For this review, take the finished solid that the model builds, in its own axes (mm). Round coordinates to 2 decimals unless told otherwise and drop trailing zeros. Loops run counter-clockwise (first coordinate to the right, second up) from the corner with the lowest first, then second, coordinate; pieces in that order, holes last. Notation, with made-up numbers: (-20.75, 28) -> (19.25, 28) arc R26 cw to (19.25, 46) -> close; hole circle Ø1 at (-9, -23.75). An arc over 180 degrees is marked (long way). One line per question, with ' | ' between items. Start each with the question number.
1. Consider section B-B (z = -61). Write out the cut boundary in (x, y).
2. Consider section A-A (z = -15). Write out the cut boundary in (x, y), and give its area (4 significant figures).
3. For pin 1 Ø4 at (x, z) = (0, -15) entering from +Y, flat-tipped, find the tip position at first contact; note if it passes through.
4. Consider section C-C (y = 3.25). Count the separate pieces of the cut face and the enclosed holes in it, and give its area (3 significant figures).
5. Wall thickness on line 1 along X through (y, z) = (4.45, -33); line 2 along Z through (x, y) = (0, 1.2); line 3 along X through (y, z) = (3.95, -31): over which ranges is each line inside the solid? List them lowest first.
6. Consider section D-D (z = 55). Write out the cut boundary in (x, y).
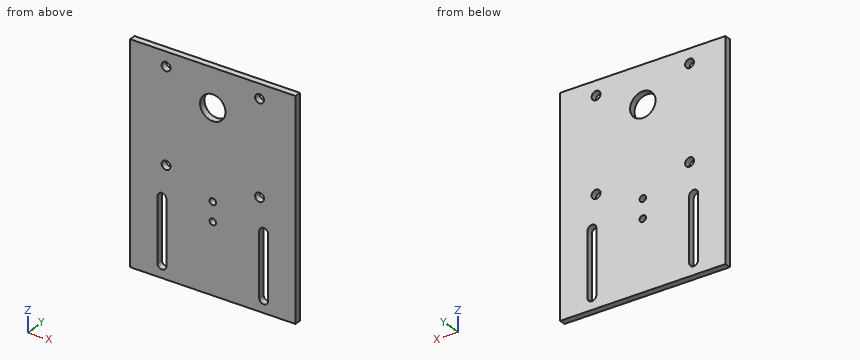
```python
from build123d import *

# Parameters (mm, degrees)
SKETCH_3_W          = 130
SKETCH_3_H          = 170
EXTRUDE_1_DEPTH     = 5
SKETCH_4_R          = 10
CUT_EXTRUDE_1_DEPTH = 10
SKETCH_5_R          = 3.5
SKETCH_5_R_2        = 2.55
CUT_EXTRUDE_2_DEPTH = 10


with BuildPart() as part:
    # 草图3 → 凸台-拉伸1 (new body)
    with BuildSketch(Plane(origin=(0, 0, 0), x_dir=(1, 0, 0), z_dir=(0, 1, 0))):
        Rectangle(SKETCH_3_W, SKETCH_3_H)
    extrude(amount=EXTRUDE_1_DEPTH)

    # 草图4 → 切除-拉伸1 (cut)
    with BuildSketch(Plane.XZ):
        with Locations((0, 55)):
            Circle(SKETCH_4_R)
    extrude(amount=-CUT_EXTRUDE_1_DEPTH, mode=Mode.SUBTRACT)

    # 草图5 → 切除-拉伸2 (cut)
    with BuildSketch(Plane.XZ):
        with Locations((36.769552622, 0.230447378)):
            Circle(SKETCH_5_R)
        with Locations((-36.769552622, 0.230447378)):
            Circle(SKETCH_5_R)
        with Locations((-36.769552622, 73.769552622)):
            Circle(SKETCH_5_R)
        with Locations((36.769552622, 73.769552622)):
            Circle(SKETCH_5_R)
        with Locations((0, -30)):
            Circle(SKETCH_5_R_2)
        with Locations((0, -15)):
            Circle(SKETCH_5_R_2)
        with BuildLine():
            Line((36.5, -75), (36.5, -25))
            ThreePointArc((36.5, -25), (40, -21.5), (43.5, -25))
            Line((43.5, -25), (43.5, -75))
            ThreePointArc((43.5, -75), (40, -78.5), (36.5, -75))
        make_face()
        with BuildLine():
            Line((-36.5, -75), (-36.5, -25))
            ThreePointArc((-36.5, -25), (-40, -21.5), (-43.5, -25))
            Line((-43.5, -25), (-43.5, -75))
            ThreePointArc((-43.5, -75), (-40, -78.5), (-36.5, -75))
        make_face()
    extrude(amount=-CUT_EXTRUDE_2_DEPTH, mode=Mode.SUBTRACT)


solid = part.part
```
Answer block:
1) outline: (-65, 0) -> (-43.5, 0) -> (-43.5, 5) -> (-65, 5) -> close; (-36.5, 0) -> (36.5, 0) -> (36.5, 5) -> (-36.5, 5) -> close; (43.5, 0) -> (65, 0) -> (65, 5) -> (43.5, 5) -> close
2) outline: (-65, 0) -> (-2.55, 0) -> (-2.55, 5) -> (-65, 5) -> close; (2.55, 0) -> (65, 0) -> (65, 5) -> (2.55, 5) -> close | area: 624.5 mm2
3) pin 1: passes through
4) separate pieces: 1 | enclosed holes: 9 | area: 20,800 mm2
5) line 1: x = -65 to -43.5, -36.5 to 36.5, 43.5 to 65 | line 2: z = -85 to -32.55, -27.45 to -17.55, -12.45 to 45, 65 to 85 | line 3: x = -65 to -43.5, -36.5 to -2.35, 2.35 to 36.5, 43.5 to 65
6) outline: (-65, 0) -> (-10, 0) -> (-10, 5) -> (-65, 5) -> close; (10, 0) -> (65, 0) -> (65, 5) -> (10, 5) -> close
